Source: CAD feature listing. Evaluate the final solid. Frame: model axes, mm. Face numbers are marked on the shaded views. A direction names the side the tool comes from. Give positions to 0.01 mm unless a question says otherwise; leave off trailing zeros. Loops run counter-clockwise (first coordinate to the right, second up) from the corner with the lowest first, then second, coordinate; pieces in that order, holes last.
from build123d import *

# Parameters (mm, degrees)
BOSS_EXTRUDE2_DEPTH  = 12
BOSS_EXTRUDE3_DEPTH  = 17
MIRROR12_DEPTH       = 29
MIRROR12_2_OUTLINE_R = 6
MIRROR12_2_DEPTH     = 12
SKETCH4_R            = 21.05
CUT_EXTRUDE1_DEPTH   = 12
SKETCH5_R            = 18.6
CUT_EXTRUDE2_DEPTH   = 5


# Read off the part's stored shape, not the designer's step: Mirror12
with BuildPart() as part:
    # Sketch1 → Boss-Extrude2 (new body)
    with BuildSketch(Plane(origin=(0, 0, 0), x_dir=(1, 0, 0), z_dir=(0, 1, 0))):
        with BuildLine():
            Line((0, 30), (0, 0))
            Line((0, 0), (39, 0))
            ThreePointArc((39, 0), (45, 6), (51, 0))
            Line((51, 0), (56.5, 0))
            ThreePointArc((56.5, 0), (54.959292144, 5.75), (50.75, 9.959292144))
            Line((50.75, 9.959292144), (21.213203436, 21.213203436))
            ThreePointArc((21.213203436, 21.213203436), (11.480502971, 27.716385975), (0, 30))
        make_face()
    extrude(amount=BOSS_EXTRUDE2_DEPTH)

    # Sketch3 → Boss-Extrude3 (add)
    with BuildSketch(Plane(origin=(0, 12, 0), x_dir=(1, 0, 0), z_dir=(0, 1, 0))):
        with BuildLine():
            Line((0, 30), (0, 0))
            Line((0, 0), (30, 0))
            ThreePointArc((30, 0), (21.213203436, 21.213203436), (0, 30))
        make_face()
    extrude(amount=BOSS_EXTRUDE3_DEPTH)

    # Mirror12 outline → Mirror12 (add)
    with BuildSketch(Plane(origin=(0, 0, 0), x_dir=(1, 0, 0), z_dir=(0, 1, 0))):
        with BuildLine():
            ThreePointArc((0, 30), (-21.213203436, -21.213203436), (30, 0))
            Line((30, 0), (0, 0))
            Line((0, 0), (0, 30))
        make_face()
    extrude(amount=MIRROR12_DEPTH)

    # Mirror12 2 outline → Mirror12 2 (add)
    # profile 1 of 2: a face of its own
    with BuildSketch(Plane(origin=(0, 0, 0), x_dir=(1, 0, 0), z_dir=(0, 1, 0))):
        with BuildLine():
            Line((56.5, 0), (51, 0))
            ThreePointArc((51, 0), (45, -6), (39, 0))
            Line((39, 0), (30, 0))
            ThreePointArc((30, 0), (27.716385975, -11.480502971), (21.213203436, -21.213203436))
            Line((21.213203436, -21.213203436), (50.75, -9.959292144))
            ThreePointArc((50.75, -9.959292144), (54.959292144, -5.75), (56.5, 0))
        make_face()
    # profile 2 of 2: a face of its own
    with BuildSketch(Plane(origin=(0, 0, 0), x_dir=(1, 0, 0), z_dir=(0, 1, 0))):
        with BuildLine():
            ThreePointArc((-21.213203436, -21.213203436), (-30, 0), (-21.213203436, 21.213203436))
            Line((-21.213203436, 21.213203436), (-50.75, 9.959292144))
            ThreePointArc((-50.75, 9.959292144), (-56.5, 0), (-50.75, -9.959292144))
            Line((-50.75, -9.959292144), (-21.213203436, -21.213203436))
        make_face()
        with Locations((-45, 0)):
            Circle(MIRROR12_2_OUTLINE_R, mode=Mode.SUBTRACT)
    extrude(amount=MIRROR12_2_DEPTH)

    # Sketch4 → Cut-Extrude1 (cut)
    with BuildSketch(Plane(origin=(0, 29, 0), x_dir=(1, 0, 0), z_dir=(0, 1, 0))):
        with Locations(Location((0, 0, 0), (0, 0, 270))):
            Circle(SKETCH4_R)
    cut_extrude1 = extrude(amount=-CUT_EXTRUDE1_DEPTH, mode=Mode.SUBTRACT)

    # Mirror13: Cut-Extrude1 across plane
    add(cut_extrude1.mirror(Plane.ZX.offset(14.5)), mode=Mode.SUBTRACT)

    # Sketch5 → Cut-Extrude2 (cut)
    with BuildSketch(Plane(origin=(0, 17, 0), x_dir=(1, 0, 0), z_dir=(0, 1, 0))):
        with Locations(Location((0, 0, 0), (0, 0, 270))):
            Circle(SKETCH5_R)
    extrude(amount=-CUT_EXTRUDE2_DEPTH, mode=Mode.SUBTRACT)


solid = part.part
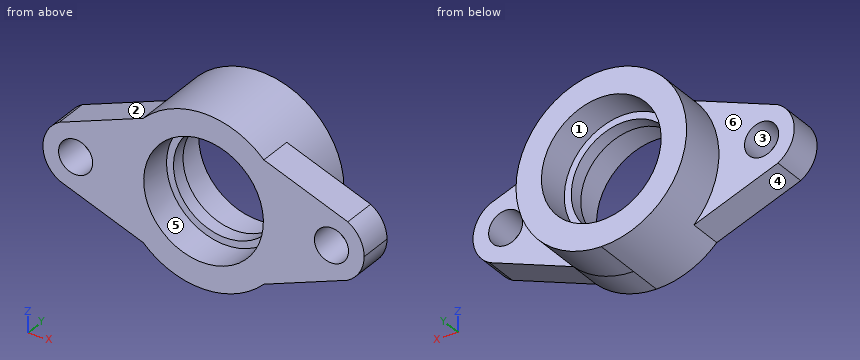
1) Cut plane D-D (y = 19.75). Return loops of the section in (x, z).
Checks:
outline: circle Ø60 at (0, 0); hole circle Ø42.1 at (0, 0)
2) Pull-direction query (X, two-part tool) for the marked faces 3, 4, 5 and 6; classes: released by +X, released by -X, zero draft, split by the parting line, or undercut.
Checks:
face 3: undercut
face 4: released by -X
face 5: undercut
face 6: zero draft
3) Cut plane B-B (y = 8). Return loops of the section in (x, z).
Checks:
outline: (-50.75, -9.96) - (-21.21, -21.21) arc R30 ccw to (21.21, -21.21) - (50.75, -9.96) arc R11.5 ccw to (50.75, 9.96) - (21.21, 21.21) arc R30 ccw to (-21.21, 21.21) - (-50.75, 9.96) arc R11.5 ccw to start; hole circle Ø12 at (-45, 0); hole circle Ø42.1 at (0, 0); hole circle Ø12 at (45, 0)
4) Cut plane A-A (x = -8). Return loops of the section in (y, z).
Checks:
outline: (0, -28.91) - (29, -28.91) - (29, -19.47) - (17, -19.47) - (17, -16.79) - (12, -16.79) - (12, -19.47) - (0, -19.47) - close; (0, 19.47) - (12, 19.47) - (12, 16.79) - (17, 16.79) - (17, 19.47) - (29, 19.47) - (29, 28.91) - (0, 28.91) - close
5) Contact query for flat-ended pins moving along their axis: P1, Ø12, axis at y = 25, z = 10.5, coming from the -X side; P2, Ø2, axis at y = 25, z = 3.5, coming from the +X side; P3, Ø10.5, axis at x = -46, z = -5.5, coming from the +Y side; P4, Ø9.5, axis at x = -45, z = 0, coming from the -Y side. Output: stop coordinate, or through.
Checks:
P1: stops at x = -29.66
P2: stops at x = 29.9
P3: stops at y = 12
P4: passes through
6) Ray query, probe 1 along X at (y, z) = (13.1, 0); probe 2 along X at (y, z) = (9, 3.5); probe 3 along X at (y, z) = (25.75, 0). Return the intervals inside material, ascending.
Checks:
probe 1: x = -30 to -18.6, 18.6 to 30
probe 2: x = -55.95 to -49.87, -40.13 to -20.76, 20.76 to 40.13, 49.87 to 55.95
probe 3: x = -30 to -21.05, 21.05 to 30
7) Reachability of the marked faces 1 and 2 from +Z, -Z, +X, -X, +Y, -Y: full face, straight path, thin tool, end or side. Return the list, or none.
Checks:
face 1: +Y
face 2: +Z, -X, +Y, -Y
8) Cut plane C-C (z = -16). Return loops of the section in (x, y).
Checks:
outline: (-34.9, 0) - (-13.68, 0) - (-13.68, 12) - (-9.48, 12) - (-9.48, 17) - (-13.68, 17) - (-13.68, 29) - (-25.38, 29) - (-25.38, 12) - (-34.9, 12) - close; (9.48, 12) - (13.68, 12) - (13.68, 0) - (34.9, 0) - (34.9, 12) - (25.38, 12) - (25.38, 29) - (13.68, 29) - (13.68, 17) - (9.48, 17) - close
